from build123d import *

# Parameters (mm, degrees)
SKETCH_1_W         = 25
SKETCH_1_H         = 8
EXTRUDE_1_DEPTH    = 4
HOLE_WIZARD_M3_1_D = 2.5
HOLE_WIZARD_M3_2_D = 2.5
CHAMFER_1_SIZE     = 0.2


with BuildPart() as part:
    # 草图1 → 凸台-拉伸1 (new, symmetric)
    with BuildSketch(Plane(origin=(0, 0, 0), x_dir=(1, 0, 0), z_dir=(0, 1, 0))):
        Rectangle(SKETCH_1_W, SKETCH_1_H)
    extrude(amount=EXTRUDE_1_DEPTH, both=True)

    # M3 螺纹孔1 (through all)
    with Locations(Plane(origin=(0, 4, 0), x_dir=(1, 0, 0), z_dir=(0, 1, 0))):
        with Locations((-7.5, 0), (2.5, 0)):
            Hole(HOLE_WIZARD_M3_1_D / 2)

    # M3 螺纹孔2 (through all)
    with Locations(Plane(origin=(0, 0, -4), x_dir=(-1, 0, 0), z_dir=(0, 0, -1))):
        with Locations((-7.5, 0), (2.5, 0)):
            Hole(HOLE_WIZARD_M3_2_D / 2)

    # 倒角1
    chamfer_1_edges = [part.edges().sort_by_distance(p)[0] for p in [
        (-12.5, 4, 0),
        (3.75, 4, 0),
        (3.75, -4, 0),
        (0, 4, 4),
        (-6.25, 4, 0),
        (-6.25, -4, 0),
        (-3.75, 0, -4),
        (-3.75, 0, 4),
        (6.25, 0, -4),
        (6.25, 0, 4),
        (12.5, 4, 0),
        (0, -4, 4),
        (-12.5, -4, 0),
        (0, -4, -4),
        (12.5, -4, 0),
        (12.5, 0, 4),
        (-12.5, 0, 4),
        (-12.5, 0, -4),
        (12.5, 0, -4),
        (0, 4, -4),
    ]]
    chamfer(chamfer_1_edges, length=CHAMFER_1_SIZE)


solid = part.part
Source: CAD feature listing. Evaluate the final solid. Frame: model axes, mm. Round coordinates to 2 decimals unless told otherwise and drop trailing zeros. Write each loop counter-clockwise with the first axis right and the second up, starting at its lowest first coordinate (ties: lowest second). Pieces come first, ordered by that corner, then holes. Notation, with made-up numbers: (-22, 73.5) - (37, 73.5) arc R19 cw to (37, 77.5) - close; hole circle Ø10 at (66.25, 67). An arc over 180 degrees is marked (long way). Use CSV: the item, a comma, the result in double quotes. Start each with the question number.
(1) Cut plane D-D, the plane z = 1.75. Return loops of the section in (x, y).
(2) Mould query, pull axis Y, two halves, no side actions, for faces 1 (the face through (0, 0, 4)), 2 (the face through (0, -4, 0)), 3 (the face through (6.25, 0.05, 0.05)). Classes: pulls with the +Y half, pulls with the -Y half, needs draft (parallel to the pull), parting line crosses it, or undercut.
(3) Cut plane A-A, the plane z = 0. Return loops of the section in (x, y).
(4) Cut plane B-B, the plane y = 3. Return loops of the section in (x, z), and give its area (3 significant figures).
(5) Cut plane C-C, the plane x = 2.5. Return loops of the section in (y, z), and give its area (3 significant figures).
(6) Material intervals for probe 1 along X at (y, z) = (-2, 0); probe 2 along Z at (x, y) = (-7.5, -2.5), sorted ascending. Write a range as [from, to].
Geometry says:
1,outline,"(-12.5, -3.8) - (-12.3, -4) - (12.3, -4) - (12.5, -3.8) - (12.5, 3.8) - (12.3, 4) - (-12.3, 4) - (-12.5, 3.8) - close; hole circle Ø2.5 at (-2.5, 0); hole circle Ø2.5 at (7.5, 0)"
2,face 1,"needs draft"
2,face 2,"pulls with the -Y half"
2,face 3,"undercut"
3,outline,"(-12.5, -3.8) - (-12.3, -4) - (-8.95, -4) - (-8.75, -3.8) - (-8.75, 3.8) - (-8.95, 4) - (-12.3, 4) - (-12.5, 3.8) - close; (-6.25, -3.8) - (-6.05, -4) - (1.05, -4) - (1.25, -3.8) - (1.25, 3.8) - (1.05, 4) - (-6.05, 4) - (-6.25, 3.8) - close; (3.75, -3.8) - (3.95, -4) - (12.3, -4) - (12.5, -3.8) - (12.5, 3.8) - (12.3, 4) - (3.95, 4) - (3.75, 3.8) - close; hole circle Ø2.5 at (-2.5, 0); hole circle Ø2.5 at (7.5, 0)"
4,outline,"(-12.5, -3.8) - (-12.3, -4) - (12.3, -4) - (12.5, -3.8) - (12.5, 3.8) - (12.3, 4) - (-12.3, 4) - (-12.5, 3.8) - close; hole circle Ø2.5 at (-7.5, 0); hole circle Ø2.5 at (2.5, 0)"
4,area,"190 mm²"
5,outline,"(-4, -3.8) - (-3.8, -4) - (3.8, -4) - (4, -3.8) - (4, -1.45) - (3.8, -1.25) - (-3.8, -1.25) - (-4, -1.45) - close; (-4, 1.45) - (-3.8, 1.25) - (3.8, 1.25) - (4, 1.45) - (4, 3.8) - (3.8, 4) - (-3.8, 4) - (-4, 3.8) - close"
5,area,"43.8 mm²"
6,probe 1,"[-12.5, -8.75], [-6.25, 1.25], [3.75, 12.5]"
6,probe 2,"[-4, -1.25], [1.25, 4]"
